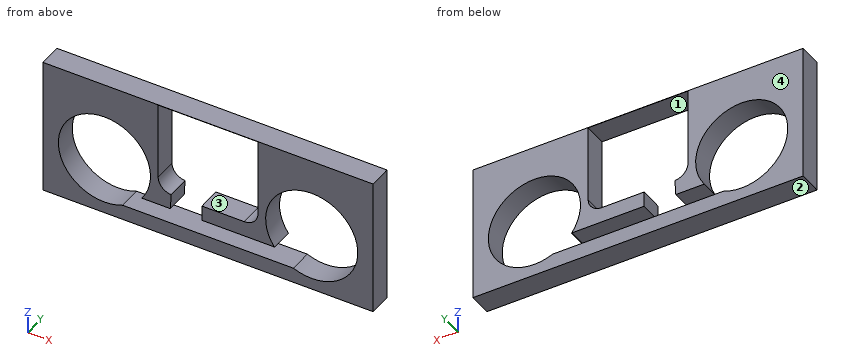
from build123d import *

# Parameters (mm, degrees)
F0_W     = 273.05
F0_H     = 114.3
F1_DEPTH = 19.05
F2_R     = 38.1
F3_DEPTH = 25.4
F5_DEPTH = 25.4
F6_DEPTH = 25.4
F8_DEPTH = 25.4


with BuildPart() as f1:
    # F0 (on Front) → F1 (new body)
    with BuildSketch(Plane.XZ):
        with Locations((136.525, 57.15)):
            Rectangle(F0_W, F0_H)
    extrude(amount=F1_DEPTH)

    # F2 (on Front) → F3 (cut)
    with BuildSketch(Plane.XZ):
        with Locations((50.8, 47.625)):
            Circle(F2_R)
        with Locations((222.25, 47.625)):
            Circle(F2_R)
    extrude(amount=F3_DEPTH, mode=Mode.SUBTRACT)

    # F4 (on Front) → F5 (cut)
    with BuildSketch(Plane.XZ):
        with BuildLine():
            Line((177.8, 114.074679), (95.25, 114.074679))
            Line((95.25, 114.074679), (95.25, 49.53))
            ThreePointArc((95.25, 49.53), (98.597769, 41.447769), (106.68, 38.1))
            Line((106.68, 38.1), (166.37, 38.1))
            ThreePointArc((166.37, 38.1), (174.452231, 41.447769), (177.8, 49.53))
            Line((177.8, 49.53), (177.8, 114.074679))
        make_face()
    extrude(amount=-F5_DEPTH, mode=Mode.SUBTRACT)

    # F4 (on Front) → F6 (cut)
    with BuildSketch(Plane.XZ):
        with BuildLine():
            Line((177.8, 114.074679), (95.25, 114.074679))
            Line((95.25, 114.074679), (95.25, 49.53))
            ThreePointArc((95.25, 49.53), (98.597769, 41.447769), (106.68, 38.1))
            Line((106.68, 38.1), (166.37, 38.1))
            ThreePointArc((166.37, 38.1), (174.452231, 41.447769), (177.8, 49.53))
            Line((177.8, 49.53), (177.8, 114.074679))
        make_face()
    extrude(amount=F6_DEPTH, mode=Mode.SUBTRACT)

    # F7 (on Front) → F8 (cut)
    with BuildSketch(Plane.XZ):
        Polygon((131.474693, 38.327217), (106.074693, 38.327217), (105.311239, 25.348496), (79.911239, 25.348496), (50.899979, 12.648496), (220.386818, 12.648496), (190.993831, 25.348496), (131.474693, 25.348496), align=None)
    extrude(amount=F8_DEPTH, mode=Mode.SUBTRACT)


solid = f1.part
Geometry: final body of the model. Coordinates: model frame, mm. Face numbers are marked on the shaded views. A direction names the side the tool comes from. Give positions to 0.01 mm unless a question says otherwise; leave off trailing zeros. Loops run counter-clockwise (first coordinate to the right, second up) from the corner with the lowest first, then second, coordinate; pieces in that order, holes last. Notation, with made-up numbers: (-23.75, 55) - (-0.75, 55) arc R15 ccw to (-0.75, 75) - close; hole circle Ø9 at (33, 67). An arc over 180 degrees is marked (long way). One line per question, with ' | ' between items. Start each with the question number.
(1) Ray query, line 1 (X direction, y = -9.75, z = 48.5); line 2 (Z direction, x = 122, y = -7.75); line 3 (Z direction, x = 222.25, y = -10.25) (3 decimals). Return the intervals inside material, ascending. Write a range as from..to.
(2) Section query C-C on x = 222.25. Return loops of the section in (y, z) (3 decimals), then the cut area to 3 significant figures.
(3) Pull-direction query (X, two-part tool) for the marked faces 1 and 2; classes: released by +X, released by -X, zero draft, split by the parting line, or undercut.
(4) Section query A-A on z = 89.5. Return loops of the section in (x, y), then the cut area to 3 significant figures.
(5) Section query D-D on z = 56.5. Return loops of the section in (x, y).
(6) Reachability of the marked faces 3 and 4 from +Z, -Z, +X, -X, +Y, -Y: full face, straight path, thin tool, end or side. Return the list, or none.
The answers:
1) line 1: 0..12.71, 88.89..95.3, 177.75..184.16, 260.34..273.05 | line 2: 0..12.65, 114.07..114.3 | line 3: 0..9.525, 85.725..114.3
2) outline: (-19.05, 0) - (0, 0) - (0, 9.525) - (-19.05, 9.525) - close; (-19.05, 85.725) - (0, 85.725) - (0, 114.3) - (-19.05, 114.3) - close | area: 726 mm2
3) face 1: undercut | face 2: zero draft
4) outline: (0, -19.05) - (95.25, -19.05) - (95.25, 0) - (0, 0) - close; (177.8, -19.05) - (273.05, -19.05) - (273.05, 0) - (177.8, 0) - close | area: 3,630 mm2
5) outline: (0, -19.05) - (13.75, -19.05) - (13.75, 0) - (0, 0) - close; (87.85, -19.05) - (95.25, -19.05) - (95.25, 0) - (87.85, 0) - close; (177.8, -19.05) - (185.2, -19.05) - (185.2, 0) - (177.8, 0) - close; (259.3, -19.05) - (273.05, -19.05) - (273.05, 0) - (259.3, 0) - close
6) face 3: +Y, -Y | face 4: +Z, -Z, +X, -X, +Y
